Model file for the job. Use its own axes, mm. Coordinates: 2 decimals unless noted, no trailing zeros.
from build123d import *

# Parameters (mm, degrees)
SKETCH_R     = 1.5
SKETCH_R_2   = 2
PAD_DEPTH    = 4
CHAMFER_SIZE = 2
FILLET004_R  = 3
FILLET005_R  = 1


with BuildPart() as part:
    # Sketch → Pad (new body)
    with BuildSketch(Plane.XY):
        Polygon((0, 0), (130, 0), (130, 150), (115, 150), (0, 100), align=None)
        with Locations((5, 4)):
            Circle(SKETCH_R, mode=Mode.SUBTRACT)
        with Locations((15, 4)):
            Circle(SKETCH_R, mode=Mode.SUBTRACT)
        with Locations((25, 4)):
            Circle(SKETCH_R, mode=Mode.SUBTRACT)
        with Locations((35, 4)):
            Circle(SKETCH_R, mode=Mode.SUBTRACT)
        with Locations((45, 4)):
            Circle(SKETCH_R, mode=Mode.SUBTRACT)
        with Locations((55, 4)):
            Circle(SKETCH_R, mode=Mode.SUBTRACT)
        with Locations((65, 4)):
            Circle(SKETCH_R, mode=Mode.SUBTRACT)
        with Locations((75, 4)):
            Circle(SKETCH_R, mode=Mode.SUBTRACT)
        with Locations((85, 4)):
            Circle(SKETCH_R, mode=Mode.SUBTRACT)
        with Locations((95, 4)):
            Circle(SKETCH_R, mode=Mode.SUBTRACT)
        with Locations((105, 4)):
            Circle(SKETCH_R, mode=Mode.SUBTRACT)
        with Locations((115, 4)):
            Circle(SKETCH_R, mode=Mode.SUBTRACT)
        with Locations((125, 4)):
            Circle(SKETCH_R, mode=Mode.SUBTRACT)
        with Locations((125, 14)):
            Circle(SKETCH_R, mode=Mode.SUBTRACT)
        with Locations((125, 24)):
            Circle(SKETCH_R, mode=Mode.SUBTRACT)
        with Locations((125, 34)):
            Circle(SKETCH_R, mode=Mode.SUBTRACT)
        with Locations((125, 44)):
            Circle(SKETCH_R, mode=Mode.SUBTRACT)
        with Locations((125, 54)):
            Circle(SKETCH_R, mode=Mode.SUBTRACT)
        with Locations((125, 64)):
            Circle(SKETCH_R, mode=Mode.SUBTRACT)
        with Locations((125, 74)):
            Circle(SKETCH_R, mode=Mode.SUBTRACT)
        with Locations((125, 84)):
            Circle(SKETCH_R, mode=Mode.SUBTRACT)
        with Locations((125, 94)):
            Circle(SKETCH_R, mode=Mode.SUBTRACT)
        with Locations((125, 104)):
            Circle(SKETCH_R, mode=Mode.SUBTRACT)
        with Locations((125, 114)):
            Circle(SKETCH_R, mode=Mode.SUBTRACT)
        with Locations((125, 124)):
            Circle(SKETCH_R, mode=Mode.SUBTRACT)
        with Locations((125, 134)):
            Circle(SKETCH_R, mode=Mode.SUBTRACT)
        with Locations((125, 144)):
            Circle(SKETCH_R, mode=Mode.SUBTRACT)
        with Locations((10, 94)):
            Circle(SKETCH_R_2, mode=Mode.SUBTRACT)
        with Locations((30, 94)):
            Circle(SKETCH_R_2, mode=Mode.SUBTRACT)
        with Locations((50, 94)):
            Circle(SKETCH_R_2, mode=Mode.SUBTRACT)
        with Locations((70, 94)):
            Circle(SKETCH_R_2, mode=Mode.SUBTRACT)
        with Locations((90, 94)):
            Circle(SKETCH_R_2, mode=Mode.SUBTRACT)
        with Locations((110, 94)):
            Circle(SKETCH_R_2, mode=Mode.SUBTRACT)
    extrude(amount=PAD_DEPTH)

    # Chamfer
    chamfer_edges = [part.edges().sort_by_distance(p)[0] for p in [
        (8, 94, 4),
        (28, 94, 4),
        (48, 94, 4),
        (68, 94, 4),
        (88, 94, 4),
        (108, 94, 4),
    ]]
    chamfer(chamfer_edges, length=CHAMFER_SIZE)

    # Fillet004
    fillet004_edges = [part.edges().sort_by_distance(p)[0] for p in [
        (0, 0, 2),
        (0, 100, 2),
        (130, 0, 2),
        (130, 150, 2),
    ]]
    fillet(fillet004_edges, radius=FILLET004_R)

    # Fillet005
    fillet005_edges = [part.edges().sort_by_distance(p)[0] for p in [
        (130, 75, 0),
        (130, 3, 2),
        (130, 147, 2),
        (130, 75, 4),
    ]]
    fillet(fillet005_edges, radius=FILLET005_R)


solid = part.part
Q1. Mould opens along Y. For faces 1 (the face through (123.5, 24.07, 1.97)), 2 (the face through (10, 96, 1)), 3 (the face through (59.194, 125.737, 1.986)) say: pulls with the +Y half, pulls with the -Y half, needs draft (parallel to the pull), parting line crosses it, or undercut.
Established:
face 1: undercut
face 2: undercut
face 3: pulls with the +Y half
Q2. Drop flat-ended pins along their axis: P1, Ø4, axis at x = 115, y = 4, coming from the +Z side; P2, Ø1.8, axis at x = 5, y = 4, coming from the +Z side; P3, Ø1, axis at x = 108.5, z = 1, coming from the +Y side; P4, Ø1.5, axis at x = 93.5, z = 1, coming from the +Y side. Give the stop position or say it passes through.
Established:
P1: stops at z = 4
P2: passes through
P3: stops at y = 147.39
P4: stops at y = 140.98
Q3. Probe line 1 (X direction, y = 64, z = 2.65); line 2 (Y direction, x = 115, z = 1.7); line 3 (Y direction, x = 35, z = 2). List the from-to ranges inside material, lowest first.
Established:
line 1: x = 0 to 123.5, 126.5 to 130
line 2: y = 0 to 2.5, 5.5 to 150
line 3: y = 0 to 2.5, 5.5 to 115.22
